Source: three-view drawing plus pictorial views. Frame: mm from the lowest corner of the part. A direction names the side the tool comes from. Coordinates: 2 decimals unless noted, no trailing zeros. Write each loop counter-clockwise with the first axis right and the second up, starting at its lowest first coordinate (ties: lowest second). Pieces come first, ordered by that corner, then holes.
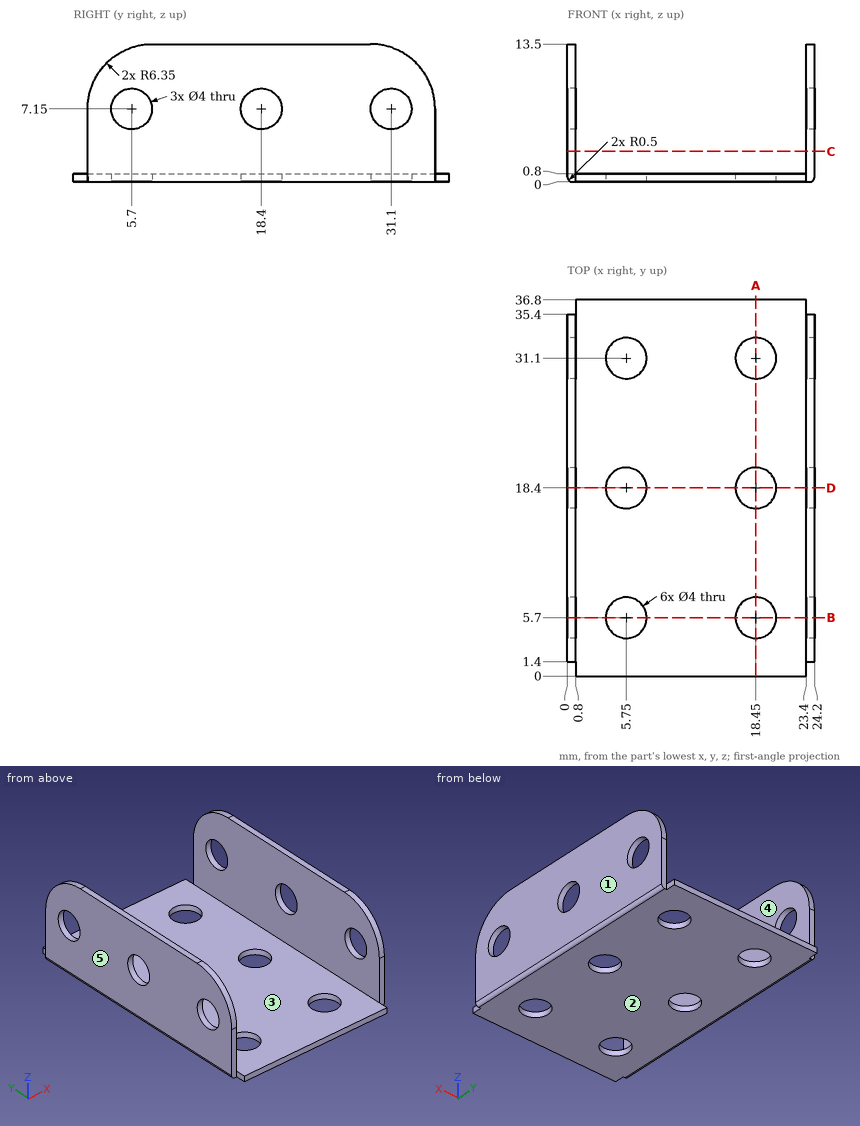
Item 1: Pull-direction query (X, two-part tool) for the marked faces 1, 2 and 3; classes: released by +X, released by -X, zero draft, split by the parting line, or undercut.
Item 2: Section query A-A, the plane x = 18.45. Return loops of the section in (y, z).
Item 3: Section query B-B, the plane y = 5.7. Return loops of the section in (x, z), then the cut area to 3 significant figures.
Item 4: Material intervals for line 1 (Y direction, x = 5.75, z = 0.3); line 2 (X direction, y = 11, z = 11.75); line 3 (Z direction, x = 22, y = 6), sorted ascending.
Item 5: Pin query (flat end, axial travel): pin 1 Ø0.6 at (x, z) = (0.5, 2.5) entering from +Y; pin 2 Ø5 at (y, z) = (5.7, 7.15) entering from -X; pin 3 Ø3.5 at (x, y) = (18.45, 18.4) entering from -Z; pin 4 Ø11.5 at (x, y) = (10, 14) entering from +Z. Return the tip coordinate at first contact, or that it passes through.
Item 6: Section query D-D, the plane y = 18.4. Return loops of the section in (x, z), then the cut area to 3 significant figures.
Item 7: Access query for the marked faces 4 and 5. Directions: +Z, -Z, +X, -X, +Y, -Y. A direction counts if a zero-diameter tool reaches every point of the face in a straight line with its end or side. Return the directions, or none.
Item 8: Section query C-C, the plane z = 3. Return loops of the section in (x, y), then the cut area to 3 significant figures.
The answers:
1. face 1: released by +X
1. face 2: zero draft
1. face 3: undercut
2. outline: (0, 0) - (3.7, 0) - (3.7, 0.8) - (0, 0.8) - close; (7.7, 0) - (16.4, 0) - (16.4, 0.8) - (7.7, 0.8) - close; (20.4, 0) - (29.1, 0) - (29.1, 0.8) - (20.4, 0.8) - close; (33.1, 0) - (36.8, 0) - (36.8, 0.8) - (33.1, 0.8) - close
3. outline: (0, 0.5) arc R0.5 ccw to (0.5, 0) - (3.75, 0) - (3.75, 0.8) - (0.8, 0.8) - (0.8, 5.15) - (0, 5.15) - close; (0, 9.15) - (0.8, 9.15) - (0.8, 13.16) - (0, 13.16) - close; (7.75, 0) - (16.45, 0) - (16.45, 0.8) - (7.75, 0.8) - close; (20.45, 0) - (23.7, 0) arc R0.5 ccw to (24.2, 0.5) - (24.2, 5.15) - (23.4, 5.15) - (23.4, 0.8) - (20.45, 0.8) - close; (23.4, 9.15) - (24.2, 9.15) - (24.2, 13.16) - (23.4, 13.16) - close
3. area: 26.2 mm2
4. line 1: y = 0 to 3.7, 7.7 to 16.4, 20.4 to 29.1, 33.1 to 36.8
4. line 2: x = 0 to 0.8, 23.4 to 24.2
4. line 3: z = 0 to 0.8
5. pin 1: stops at y = 35.4
5. pin 2: stops at x = 0
5. pin 3: passes through
5. pin 4: stops at z = 0.8
6. outline: (0, 0.5) arc R0.5 ccw to (0.5, 0) - (3.75, 0) - (3.75, 0.8) - (0.8, 0.8) - (0.8, 5.15) - (0, 5.15) - close; (0, 9.15) - (0.8, 9.15) - (0.8, 13.5) - (0, 13.5) - close; (7.75, 0) - (16.45, 0) - (16.45, 0.8) - (7.75, 0.8) - close; (20.45, 0) - (23.7, 0) arc R0.5 ccw to (24.2, 0.5) - (24.2, 5.15) - (23.4, 5.15) - (23.4, 0.8) - (20.45, 0.8) - close; (23.4, 9.15) - (24.2, 9.15) - (24.2, 13.5) - (23.4, 13.5) - close
6. area: 26.8 mm2
7. face 4: +Z, +Y, -Y
7. face 5: +Z, -Z, -X, +Y, -Y
8. outline: (0, 1.4) - (0.8, 1.4) - (0.8, 35.4) - (0, 35.4) - close; (23.4, 1.4) - (24.2, 1.4) - (24.2, 35.4) - (23.4, 35.4) - close
8. area: 54.4 mm2
